Can you work these out from the model? Positions are in its coordinate system, mm. A direction names the side the tool comes from. Round coordinates to 2 decimals unless told otherwise and drop trailing zeros. Loops run counter-clockwise (first coordinate to the right, second up) from the corner with the lowest first, then second, coordinate; pieces in that order, holes last.
from build123d import *

# Parameters (mm, degrees)
F0_W         = 124.8456425965
F0_H         = 88.3170031011
F1_DEPTH     = 2.7760323137
F2_T1_DEPTH  = 114.4453022588
F3_T1_DEPTH  = 145.8939417542
F4_T1_DEPTH  = 109.3653022588
F5_T1_DEPTH  = 140.8139417542
F6_R         = 5.08
F7_T1_DEPTH  = 56.8432509899
F8_T1_DEPTH  = 23.6501246691
F9_T4_DEPTH  = 47.6030598057
F10_T4_DEPTH = 72.4922642685
F11_T4_DEPTH = 72.4922642685
F12_T4_DEPTH = 74.9874005688
F13_T1_DEPTH = 41.4855244232
F14_T4_DEPTH = 109.3624946917


# Not quite as in the source:
# - a fillet or chamfer that OpenCascade refuses, or shapes differently, is made with other operations: its cross-section is extruded or revolved along the edge and cut away or added


with BuildPart() as f1:
    # F0 (on Top) → F1 (new body)
    with BuildSketch(Plane.XY):
        with Locations((2.7440618724, 2.717172727)):
            Rectangle(F0_W, F0_H)
        Polygon((-38.1721407175, -32.3632955551), (-38.1721407175, 24.4799554348), (-8.7132304907, 24.4799554348), (-8.7132304907, -16.804009676), (16.8039947748, -16.804009676), (16.8039947748, 24.4799554348), (40.4541194439, 24.4799554348), (40.4541194439, -32.3632955551), align=None, mode=Mode.SUBTRACT)
    extrude(amount=F1_DEPTH)

    # F2: chamfer of 5.08 on 1 edges, made by hand

    # F2_s2 → F2_t1 (cut)
    with BuildSketch(Plane.XZ.offset(-59.9398238564)):
        Polygon((65.1668831706, -2.3039676863), (60.0868831706, 2.7760323137), (65.1668831706, 2.7760323137), align=None)
    extrude(amount=F2_T1_DEPTH, mode=Mode.SUBTRACT)

    # F3: chamfer of 5.08 on 1 edges, made by hand

    # F3_s2 → F3_t1 (cut)
    with BuildSketch(Plane.YZ.offset(-72.7429090047)):
        Polygon((46.8756742775, -2.3039676863), (41.7956742775, 2.7760323137), (46.8756742775, 2.7760323137), align=None)
    extrude(amount=F3_T1_DEPTH, mode=Mode.SUBTRACT)

    # F4: chamfer of 5.08 on 1 edges, made by hand

    # F4_s2 → F4_t1 (cut)
    with BuildSketch(Plane.XZ.offset(-54.8598238564)):
        Polygon((-59.6787594259, -2.3039676863), (-54.5987594259, 2.7760323137), (-59.6787594259, 2.7760323137), align=None)
    extrude(amount=F4_T1_DEPTH, mode=Mode.SUBTRACT)

    # F5: chamfer of 5.08 on 1 edges, made by hand

    # F5_s2 → F5_t1 (cut)
    with BuildSketch(Plane.YZ.offset(-67.6629090048)):
        Polygon((-41.4413288236, -2.3039676863), (-36.3613288236, 2.7760323137), (-41.4413288236, 2.7760323137), align=None)
    extrude(amount=F5_T1_DEPTH, mode=Mode.SUBTRACT)

    # F6
    f6_edges = [f1.edges().sort_by_distance(p)[0] for p in [
        (2.744062, 41.795674, 2.776032),
    ]]
    fillet(f6_edges, radius=F6_R)

    # F7: chamfer of 5.08 on 1 edges, made by hand

    # F7_s2 → F7_t1 (cut)
    with BuildSketch(Plane.XZ.offset(-24.4799554348)):
        Polygon((-43.2521407175, 2.7760323137), (-38.1721407175, -2.3039676863), (-38.1721407175, 2.7760323137), align=None)
    extrude(amount=F7_T1_DEPTH, mode=Mode.SUBTRACT)

    # F8: chamfer of 5.08 on 1 edges, made by hand

    # F8_s2 → F8_t1 (cut)
    with BuildSketch(Plane.YZ.offset(16.8039947748)):
        Polygon((24.4799554348, -2.3039676863), (29.5599554348, 2.7760323137), (24.4799554348, 2.7760323137), align=None)
    extrude(amount=F8_T1_DEPTH, mode=Mode.SUBTRACT)

    # F9: chamfer of 5.08 on 1 edges, made by hand


with BuildPart() as f9_tool2:
    # F9_s3 → F9_t4 (new body)
    with BuildSketch(Plane.YZ.offset(-56.3162902964)):
        Polygon((24.4799554348, -2.3039676863), (29.5599554348, 2.7760323137), (24.4799554348, 2.7760323137), align=None)
    extrude(amount=F9_T4_DEPTH)

    split(bisect_by=Plane(origin=(-20.2380542019, 0, -20.2380542019), x_dir=(0, 1, 0), z_dir=(0.7071067812, 0, 0.7071067812)), keep=Keep.TOP)


with BuildPart() as f1_1:
    add(f1.part)

    # F9_t1: cut F9_tool2
    add(f9_tool2.part, mode=Mode.SUBTRACT)

    # F10: chamfer of 5.08 on 1 edges, made by hand


with BuildPart() as f10_tool2:
    # F10_s3 → F10_t4 (new body)
    with BuildSketch(Plane.XZ.offset(-42.6241050137)):
        Polygon((-8.7132304907, -2.3039676863), (-3.6332304907, 2.7760323137), (-8.7132304907, 2.7760323137), align=None)
    extrude(amount=F10_T4_DEPTH)

    split(bisect_by=Plane(origin=(0, 13.3919615606, -13.3919615605), x_dir=(1, 0, 0), z_dir=(0, -0.7071067812, 0.7071067812)), keep=Keep.TOP)


with BuildPart() as f1_2:
    add(f1_1.part)

    # F10_t1: cut F10_tool2
    add(f10_tool2.part, mode=Mode.SUBTRACT)

    # F11: chamfer of 5.08 on 1 edges, made by hand


with BuildPart() as f11_tool2:
    # F11_s3 → F11_t4 (new body)
    with BuildSketch(Plane.XZ.offset(29.8681592548)):
        Polygon((16.8039947748, -2.3039676863), (11.7239947748, 2.7760323137), (16.8039947748, 2.7760323137), align=None)
    extrude(amount=-F11_T4_DEPTH)

    split(bisect_by=Plane(origin=(0, 13.3919615606, -13.3919615606), x_dir=(1, 0, 0), z_dir=(0, -0.7071067812, 0.7071067812)), keep=Keep.TOP)


with BuildPart() as f1_3:
    add(f1_2.part)

    # F11_t1: cut F11_tool2
    add(f11_tool2.part, mode=Mode.SUBTRACT)

    # F12: chamfer of 5.08 on 1 edges, made by hand


with BuildPart() as f12_tool2:
    # F12_s3 → F12_t4 (new body)
    with BuildSketch(Plane.XZ.offset(-42.6241050137)):
        Polygon((40.4541194439, -2.3039676863), (45.5341194439, 2.7760323137), (40.4541194439, 2.7760323137), align=None)
    extrude(amount=F12_T4_DEPTH)

    split(bisect_by=Plane(origin=(0, 13.3919615606, -13.3919615606), x_dir=(1, 0, 0), z_dir=(0, -0.7071067812, 0.7071067812)), keep=Keep.TOP)


with BuildPart() as f1_4:
    add(f1_3.part)

    # F12_t1: cut F12_tool2
    add(f12_tool2.part, mode=Mode.SUBTRACT)

    # F13: chamfer of 5.08 on 1 edges, made by hand

    # F13_s2 → F13_t1 (cut)
    with BuildSketch(Plane.YZ.offset(-16.6973800696)):
        Polygon((-16.804009676, -2.3039676863), (-11.724009676, 2.7760323137), (-16.804009676, 2.7760323137), align=None)
    extrude(amount=F13_T1_DEPTH, mode=Mode.SUBTRACT)

    # F14: chamfer of 5.08 on 1 edges, made by hand


with BuildPart() as f14_tool2:
    # F14_s3 → F14_t4 (new body)
    with BuildSketch(Plane.YZ.offset(-53.5402579827)):
        Polygon((-37.4432955551, 0), (-32.3632955551, 5.08), (-32.3632955551, 0), align=None)
    extrude(amount=F14_T4_DEPTH)

    split(bisect_by=Plane(origin=(-20.2380542019, 0, -20.2380542019), x_dir=(0, 1, 0), z_dir=(0.7071067812, 0, 0.7071067812)), keep=Keep.TOP)

    split(bisect_by=Plane(origin=(21.3790435651, 0, -21.3790435651), x_dir=(0, 1, 0), z_dir=(-0.7071067812, 0, 0.7071067812)), keep=Keep.TOP)


with BuildPart() as f1_5:
    add(f1_4.part)

    # F14_t1: cut F14_tool2
    add(f14_tool2.part, mode=Mode.SUBTRACT)


solid = f1_5.part
(1) Will these pins go through, and if not, where does the flat tip stop? P1, Ø1, axis at x = 24, z = 1.5, coming from the -Y side; P2, Ø1, axis at y = 11, z = 2, coming from the +X side.
Worked answers:
P1: stops at y = -38.14
P2: stops at x = 61.36
(2) If we mould it in two halves opening along X, with no side actions, what happens to faces 1 (the flat face through (-41.884, -4.411, 1.407)), 2 (the flat face through (-56.006, 3.303, 1.369)), 3 (the cylindrical face through (3.57, 41.66, 2.38)), 4 (the flat face through (61.494, 3.303, 1.369))? For each: released by +X, released by -X, zero draft, split by the parting line, or undercut.
Worked answers:
face 1: undercut
face 2: released by -X
face 3: zero draft
face 4: released by +X
(3) If we section it at C-C, the plane y = -22.5: List the corners of the cut face in (x, z) for me.
Worked answers:
outline: (-57.37, 0) - (-40.48, 0) - (-43.25, 2.78) - (-54.6, 2.78) - close; (42.76, 0) - (62.86, 0) - (60.09, 2.78) - (45.53, 2.78) - close
(4) If we section it at D-D, the plane z = 0.5: List the corners of the cut face in (x, y) for me.
Worked answers:
outline: (-56.87, -38.64) - (62.36, -38.64) - (62.36, 44.07) - (-56.87, 44.07) - close; hole (-40.98, -36.94) - (43.26, -36.94) - (43.26, 27.28) - (14, 27.28) - (14, -14) - (-5.91, -14) - (-5.91, 27.28) - (-40.98, 27.28) - close
(5) If I drill on line 1 (X direction, y = -12.5, z = 1.55); line 2 (X direction, y = -7.5, z = 0.9); line 3 (Y direction, x = 8, z = 1.95), over which ranges is the centre line in solid material (lowest first)?
Worked answers:
line 1: x = -55.82 to -42.03, -4.86 to 12.95, 44.31 to 61.31
line 2: x = -56.47 to -41.38, -5.51 to 13.6, 43.66 to 61.96
line 3: y = -37.19 to -35.49, -12.55 to 42.47
(6) If we section it at B-B, the plane y = -6: List the corners of the cut face in (x, z) for me, then the cut area to 3 significant figures.
Worked answers:
outline: (-57.37, 0) - (-40.48, 0) - (-43.25, 2.78) - (-54.6, 2.78) - close; (-6.41, 0) - (14.5, 0) - (11.72, 2.78) - (-3.63, 2.78) - close; (42.76, 0) - (62.86, 0) - (60.09, 2.78) - (45.53, 2.78) - close
area: 138 mm2
(7) If we section it at A-A, the plane x = 5.5: List the corners of the cut face in (y, z) for me.
Worked answers:
outline: (-39.14, 0) - (-37.44, 0) - (-34.67, 2.78) - (-36.36, 2.78) - close; (-14.5, 0) - (44.57, 0) - (43.28, 1.29) arc R5.08 ccw to (39.69, 2.78) - (-11.72, 2.78) - close
(8) For faces 5 (the flat face through (1.9, -37.77, 1.37)), 6 (the flat face through (28.392, 28.191, 1.407)), which set-ups out of +Z, -Z, +X, -X, +Y, -Y let a thin tool reach every point of the face, with its end or its side?
Worked answers:
face 5: +Z, +X, -X, -Y
face 6: +Z
